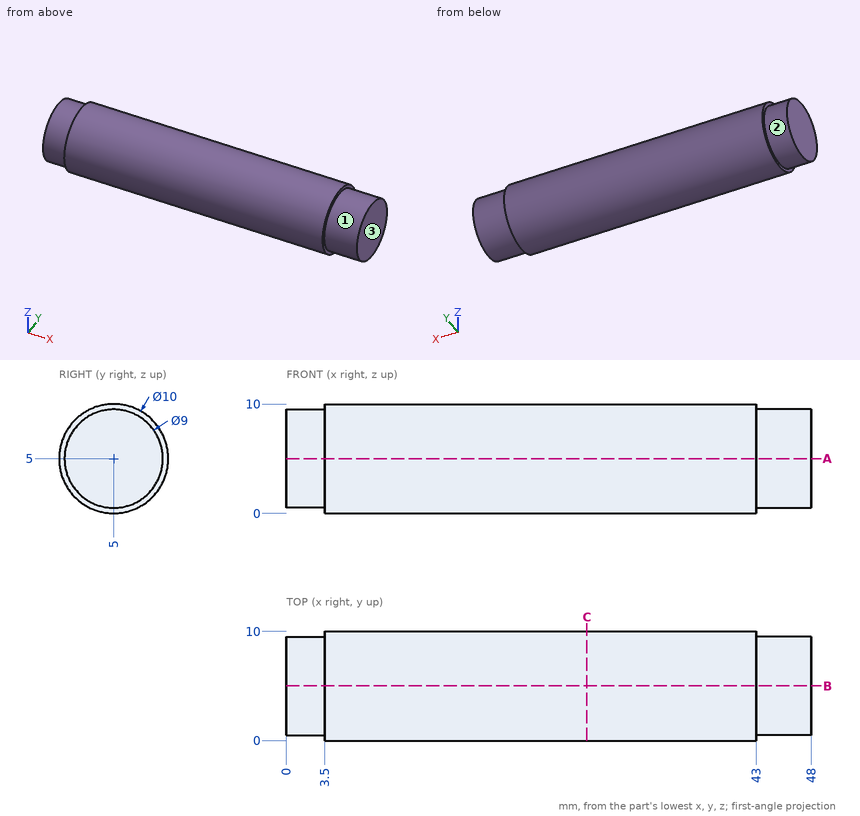
Could you check a few things on this drawing? It's one solid part, dimensions in mm from its lowest x, y, z. A direction names the side the tool comes from. Round coordinates to 2 decimals unless told otherwise and drop trailing zeros. Order: outer loops, then holes, each group sorted by start corner. A loop starts at its lowest first (then second) coordinate and runs counter-clockwise, first axis right, second up. Notation, with made-up numbers: M 18.25,-32.75 L 66.25,-32.75 A14 ccw 66.25,-24.75 Z; hole C 89,-22 d4. An arc over 180 degrees is marked long. One line per question, with ' | ' between items.
1) I'm going to push flat-ended pins straight in: pin 1 Ø1.5 at (x, y) = (30, 8.5) entering from -Z; pin 2 Ø2 at (x, z) = (6.5, 1.5) entering from -Y; pin 3 Ø2 at (x, y) = (42, 3.5) entering from +Z. Where does each tip first touch, or does it pass through?
Checked values:
pin 1: stops at z = 0.82 | pin 2: stops at y = 0.67 | pin 3: stops at z = 9.97
2) On a 3-axis mill with a long thin cutter (end or side, diameter ignored), from which of +Z, -Z, +X, -X, +Y, -Y can I reach the whole of each face in a straight line? I mean the marked faces 1, 2 and 3. Say none if no direction works.
Checked values:
face 1: +X | face 2: -X | face 3: +Z, -Z, +X, +Y, -Y
3) Imagine slicing it at C-C, the plane x = 27.5. Write out the boundary of the cut face in (y, z).
Checked values:
outline: C 5,5 d10
4) I need wall thicknesses on line 1 (Y direction, x = 36, z = 4.75); line 2 (Z direction, x = 45.5, y = 5.5); line 3 (Y direction, x = 31, z = 8). Which ranges of each line are inside material? Lowest first, please.
Checked values:
line 1: y = 0.01 to 9.99 | line 2: z = 0.53 to 9.47 | line 3: y = 1 to 9
5) Imagine slicing it at A-A, the plane z = 5. Write out the boundary of the cut face in (x, y).
Checked values:
outline: M 0,0.5 L 3.5,0.5 L 3.5,0 L 43,0 L 43,0.5 L 48,0.5 L 48,9.5 L 43,9.5 L 43,10 L 3.5,10 L 3.5,9.5 L 0,9.5 Z
